```python
from build123d import *

# Parameters (mm, degrees)
EXTRUDE_2_DEPTH     = 16
SKETCH_1_3_R        = 2.6
EXTRUDE_3_DEPTH     = 3
EXTRUDE_START       = 16
SKETCH_1_6_R        = 1.15
EXTRUDE_4_DEPTH     = 5
CUT_EXTRUDE_START   = 10
CUT_EXTRUDE_1_DEPTH = 13
CUT_EXTRUDE_START_2 = 12
CUT_EXTRUDE_2_DEPTH = 13
SKETCH_3_R          = 1.05
EXTRUDE_5_DEPTH     = 6
EXTRUDE_START_2     = -3
SKETCH_4_W          = 3
SKETCH_4_H          = 2.5
EXTRUDE_7_DEPTH     = 6


with BuildPart() as part:
    # 草图1 → 凸台-拉伸2 (new body)
    with BuildSketch(Plane.XY):
        with BuildLine():
            ThreePointArc((-7.141428429, 7), (-10, 0), (-7.141428429, -7))
            Line((-7.141428429, -7), (-7.141428429, -15))
            Line((-7.141428429, -15), (-4, -15))
            Line((-4, -15), (4, -15))
            Line((4, -15), (7.141428429, -15))
            Line((7.141428429, -15), (7.141428429, -7))
            ThreePointArc((7.141428429, -7), (10, 0), (7.141428429, 7))
            Line((7.141428429, 7), (7.141428429, 15))
            Line((7.141428429, 15), (15.141428429, 15))
            Line((15.141428429, 15), (15.141428429, -19.186046512))
            Line((15.141428429, -19.186046512), (-15.141428429, -19.186046512))
            Line((-15.141428429, -19.186046512), (-15.141428429, 15))
            Line((-15.141428429, 15), (-7.141428429, 15))
            Line((-7.141428429, 15), (-7.141428429, 7))
        make_face()
        with BuildLine():
            Line((-7.141428429, 4), (-7.141428429, 6))
            Line((-7.141428429, 6), (-7.141428429, 7))
            ThreePointArc((-7.141428429, 7), (-10, 0), (-7.141428429, -7))
            Line((-7.141428429, -7), (-7.141428429, -6))
            Line((-7.141428429, -6), (-7.141428429, -4))
            Line((-7.141428429, -4), (-6.194496835, -3.46961222))
            ThreePointArc((-6.194496835, -3.46961222), (-7.1, 0), (-6.194496835, 3.46961222))
            Line((-6.194496835, 3.46961222), (-7.141428429, 4))
        make_face()
        with BuildLine():
            Line((-5.234786058, 2.932066665), (-6.194496835, 3.46961222))
            ThreePointArc((-6.194496835, 3.46961222), (-7.1, 0), (-6.194496835, -3.46961222))
            Line((-6.194496835, -3.46961222), (-5.234786058, -2.932066665))
            ThreePointArc((-5.234786058, -2.932066665), (-6, 0), (-5.234786058, 2.932066665))
        make_face()
        with BuildLine():
            ThreePointArc((6.194496835, -3.46961222), (7.1, 0), (6.194496835, 3.46961222))
            Line((6.194496835, 3.46961222), (5.234786058, 2.932066665))
            ThreePointArc((5.234786058, 2.932066665), (6, 0), (5.234786058, -2.932066665))
            Line((5.234786058, -2.932066665), (6.194496835, -3.46961222))
        make_face()
        with BuildLine():
            ThreePointArc((7.141428429, -7), (10, 0), (7.141428429, 7))
            Line((7.141428429, 7), (7.141428429, 6))
            Line((7.141428429, 6), (7.141428429, 4))
            Line((7.141428429, 4), (6.194496835, 3.46961222))
            ThreePointArc((6.194496835, 3.46961222), (7.1, 0), (6.194496835, -3.46961222))
            Line((6.194496835, -3.46961222), (7.141428429, -4))
            Line((7.141428429, -4), (7.141428429, -6))
            Line((7.141428429, -6), (7.141428429, -7))
        make_face()
    extrude(amount=EXTRUDE_2_DEPTH)

    # 草图1<3> → 凸台-拉伸3 (add)
    with BuildSketch(Plane.XY):
        with BuildLine():
            Line((7.141428429, 4), (7.141428429, 6))
            Line((7.141428429, 6), (-7.141428429, 6))
            Line((-7.141428429, 6), (-7.141428429, 4))
            Line((-7.141428429, 4), (-6.194496835, 3.46961222))
            Line((-6.194496835, 3.46961222), (-5.234786058, 2.932066665))
            ThreePointArc((-5.234786058, 2.932066665), (-6, 0), (-5.234786058, -2.932066665))
            Line((-5.234786058, -2.932066665), (-6.194496835, -3.46961222))
            Line((-6.194496835, -3.46961222), (-7.141428429, -4))
            Line((-7.141428429, -4), (-7.141428429, -6))
            Line((-7.141428429, -6), (7.141428429, -6))
            Line((7.141428429, -6), (7.141428429, -4))
            Line((7.141428429, -4), (6.194496835, -3.46961222))
            Line((6.194496835, -3.46961222), (5.234786058, -2.932066665))
            ThreePointArc((5.234786058, -2.932066665), (6, 0), (5.234786058, 2.932066665))
            Line((5.234786058, 2.932066665), (6.194496835, 3.46961222))
            Line((6.194496835, 3.46961222), (7.141428429, 4))
        make_face()
        Circle(SKETCH_1_3_R, mode=Mode.SUBTRACT)
    extrude(amount=EXTRUDE_3_DEPTH)

    # 草图1<6> → 凸台-拉伸4 (add)
    # profile 1 of 2: a face of its own
    with BuildSketch(Plane.XY.offset(EXTRUDE_START)):
        with BuildLine():
            Line((-15.141428429, -2.5), (-15.141428429, 2.5))
            Line((-15.141428429, 2.5), (-20.141428429, 2.5))
            ThreePointArc((-20.141428429, 2.5), (-22.641428429, 0), (-20.141428429, -2.5))
            Line((-20.141428429, -2.5), (-15.141428429, -2.5))
        make_face()
        with Locations((-20.141428429, 0)):
            Circle(SKETCH_1_6_R, mode=Mode.SUBTRACT)
    # profile 2 of 2: a face of its own
    with BuildSketch(Plane.XY.offset(EXTRUDE_START)):
        with BuildLine():
            Line((20.141428429, 2.5), (15.141428429, 2.5))
            Line((15.141428429, 2.5), (15.141428429, -2.5))
            Line((15.141428429, -2.5), (20.141428429, -2.5))
            ThreePointArc((20.141428429, -2.5), (22.641428429, 0), (20.141428429, 2.5))
        make_face()
        with Locations((20.141428429, 0)):
            Circle(SKETCH_1_6_R, mode=Mode.SUBTRACT)
    extrude(amount=-EXTRUDE_4_DEPTH)

    # 草图1<4> → 切除-拉伸1 (cut)
    with BuildSketch(Plane.XY.offset(CUT_EXTRUDE_START)):
        with BuildLine():
            Line((-7.141428429, 4), (-7.141428429, 6))
            Line((-7.141428429, 6), (-7.141428429, 7))
            ThreePointArc((-7.141428429, 7), (-10, 0), (-7.141428429, -7))
            Line((-7.141428429, -7), (-7.141428429, -6))
            Line((-7.141428429, -6), (-7.141428429, -4))
            Line((-7.141428429, -4), (-6.194496835, -3.46961222))
            ThreePointArc((-6.194496835, -3.46961222), (-7.1, 0), (-6.194496835, 3.46961222))
            Line((-6.194496835, 3.46961222), (-7.141428429, 4))
        make_face()
        with BuildLine():
            ThreePointArc((7.141428429, -7), (10, 0), (7.141428429, 7))
            Line((7.141428429, 7), (7.141428429, 6))
            Line((7.141428429, 6), (7.141428429, 4))
            Line((7.141428429, 4), (6.194496835, 3.46961222))
            ThreePointArc((6.194496835, 3.46961222), (7.1, 0), (6.194496835, -3.46961222))
            Line((6.194496835, -3.46961222), (7.141428429, -4))
            Line((7.141428429, -4), (7.141428429, -6))
            Line((7.141428429, -6), (7.141428429, -7))
        make_face()
    extrude(amount=CUT_EXTRUDE_1_DEPTH, mode=Mode.SUBTRACT)

    # 草图1<5> → 切除-拉伸2 (cut)
    with BuildSketch(Plane.XY.offset(CUT_EXTRUDE_START_2)):
        with BuildLine():
            Line((-5.234786058, 2.932066665), (-6.194496835, 3.46961222))
            ThreePointArc((-6.194496835, 3.46961222), (-7.1, 0), (-6.194496835, -3.46961222))
            Line((-6.194496835, -3.46961222), (-5.234786058, -2.932066665))
            ThreePointArc((-5.234786058, -2.932066665), (-6, 0), (-5.234786058, 2.932066665))
        make_face()
        with BuildLine():
            ThreePointArc((6.194496835, -3.46961222), (7.1, 0), (6.194496835, 3.46961222))
            Line((6.194496835, 3.46961222), (5.234786058, 2.932066665))
            ThreePointArc((5.234786058, 2.932066665), (6, 0), (5.234786058, -2.932066665))
            Line((5.234786058, -2.932066665), (6.194496835, -3.46961222))
        make_face()
    extrude(amount=CUT_EXTRUDE_2_DEPTH, mode=Mode.SUBTRACT)

    # 草图3 → 凸台-拉伸5 (add)
    with BuildSketch(Plane(origin=(0, 0, 0), x_dir=(-1, 0, 0), z_dir=(0, 0, -1))):
        with Locations((0, 6)):
            Circle(SKETCH_3_R)
    extrude(amount=-EXTRUDE_5_DEPTH)

    # 草图4 → 凸台-拉伸7 (add)
    with BuildSketch(Plane.XY.offset(3).offset(EXTRUDE_START_2)):
        with Locations((5.5, 6.75)):
            Rectangle(SKETCH_4_W, SKETCH_4_H)
        with Locations((-5.5, 6.75)):
            Rectangle(SKETCH_4_W, SKETCH_4_H)
    extrude(amount=EXTRUDE_7_DEPTH)


solid = part.part
```
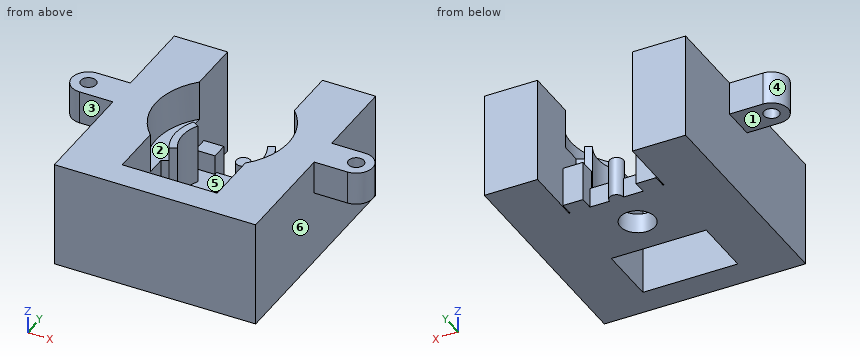
CAD build for the part. Positions are in the model's coordinates, mm. Face numbers are marked on the shaded views. A direction names the side the tool comes from. Round coordinates to 2 decimals unless told otherwise and drop trailing zeros. Write each loop counter-clockwise with the first axis right and the second up, starting at its lowest first coordinate (ties: lowest second). Pieces come first, ordered by that corner, then holes. Notation, with made-up numbers: (41, 7) -> (93, 7) arc R9 ccw to (93, 19) -> close; hole circle Ø6 at (16, -32.75). An arc over 180 degrees is marked (long way). Answer in a Markdown table with one row per item. Add a question column.
Item 1: Drop flat-ended pins along their axis: pin 1 Ø3 at (y, z) = (-3.5, 13) entering from -X; pin 2 Ø2.5 at (x, z) = (-5, 2) entering from +Y; pin 3 Ø1.5 at (y, z) = (-6, 7.5) entering from -X. Give the stop position or say it passes through.
Item 2: Which spindle directions (+Z, -Z, +X, -X, +Y, -Y) get a long thin tool onto all of the face, cutting with end or side? Do the marked faces 1, 2 and 3. Say none if no direction does.
Item 3: Saw through at C-C, the plane y = 12. Write the cut outline in (x, z).
Item 4: Saw through at D-D, the plane z = 8. Write the cut outline in (x, y), then the cut area to 3 significant figures.
Item 5: Drill centre lines: line 1 (Y direction, x = 0, z = 0.8); line 2 (X direction, y = -12, z = 5); line 3 (Z direction, x = -3, y = -1). Where is each one in solid material? Low to high. Write a range as from..to.
Item 6: Mould opens along Y. For the marked faces 4, 5 and 6 say: pulls with the +Y half, pulls with the -Y half, needs draft (parallel to the pull), parting line crosses it, or undercut.
Item 7: Saw through at A-A, the plane z = 11.5. Count the separate pieces of the cut face and the enclosed holes in it, then the cut area to 3 significant figures.
Item 8: Saw through at B-B, the plane x = 0. Write the cut outline in (y, z), then the cut area to 3 significant figures.
Findings below:
| question | item | result |
|---|---|---|
| 1 | pin 1 | stops at x = -21.64 |
| 1 | pin 2 | stops at y = 8 |
| 1 | pin 3 | stops at x = -15.14 |
| 2 | face 1 | -Z, -X, +Y, -Y |
| 2 | face 2 | +Z |
| 2 | face 3 | +Z, -Z, -X, -Y |
| 3 | outline | (-15.14, 0) -> (-7.14, 0) -> (-7.14, 16) -> (-15.14, 16) -> close; (7.14, 0) -> (15.14, 0) -> (15.14, 16) -> (7.14, 16) -> close |
| 4 | outline | (-15.14, -19.19) -> (15.14, -19.19) -> (15.14, 15) -> (7.14, 15) -> (7.14, 4) -> (5.23, 2.93) arc R6 cw to (5.23, -2.93) -> (7.14, -4) -> (7.14, -15) -> (-7.14, -15) -> (-7.14, -4) -> (-5.23, -2.93) arc R6 cw to (-5.23, 2.93) -> (-7.14, 4) -> (-7.14, 15) -> (-15.14, 15) -> close |
| 4 | area | 627 mm^2 |
| 5 | line 1 | y = -19.19..-15, -6..-2.6, 2.6..7.05 |
| 5 | line 2 | x = -15.14..-7.14, 7.14..15.14 |
| 5 | line 3 | z = 0..3 |
| 6 | face 4 | parting line crosses it |
| 6 | face 5 | undercut |
| 6 | face 6 | needs draft |
| 7 | separate pieces | 3 |
| 7 | enclosed holes | 2 |
| 7 | area | 628 mm^2 |
| 8 | outline | (-19.19, 0) -> (-15, 0) -> (-15, 16) -> (-19.19, 16) -> close; (-6, 0) -> (-2.6, 0) -> (-2.6, 3) -> (-6, 3) -> close; (2.6, 0) -> (7.05, 0) -> (7.05, 6) -> (4.95, 6) -> (4.95, 3) -> (2.6, 3) -> close |
| 8 | area | 96.8 mm^2 |
